Autodesk Inventor part; units mm, degrees
ref_plane "YZ Plane" through (0, 0, 0) normal (1, 0, 0) x (0, 1, 0)
ref_plane "XZ Plane" through (0, 0, 0) normal (0, 1, 0) x (-1, 0, 0)
ref_plane "XY Plane" through (0, 0, 0) normal (0, 0, 1) x (1, 0, 0)
sketch "Skizze1" plane through (0, 0, 0) normal (0, 0, 1) x (1, 0, 0)
  line L0 (0, -1.9) -> (0, 11.4) construction
  line L1 (-7.5, 0) -> (7.5, 0)
  line L2 (7.5, 0) -> (7.5, 9.5)
  line L3 (7.5, 9.5) -> (-7.5, 9.5)
  line L4 (-7.5, 9.5) -> (-7.5, 0)
  circle A0 centre (-7.5, 6.5) radius 1.5
  line L5 (-12.6, 0) -> (12.6, 0)
  line L6 (-4.5, 6.5) -> (-7.5, 6.5) construction
  line L7 (-4.5, 7) -> (-7.5, 7)
  line L8 (-7.5, 6) -> (-4.5, 6)
  arc A1 (-4.5, 6) -> (-4.5, 7) centre (-4.5, 6.5) ccw
  arc A2 (-7.5, 7) -> (-7.5, 6) centre (-7.5, 6.5) ccw
  circle A3 centre (-4.5, 6.5) radius 1
  circle A4 centre (7.5, 6.5) radius 1.5
  line L9 (4.5, 7) -> (7.5, 7)
  line L10 (7.5, 6) -> (4.5, 6)
  arc A5 (4.5, 7) -> (4.5, 6) centre (4.5, 6.5) ccw
  circle A6 centre (4.5, 6.5) radius 1
  point P0 (0, 0)
  point P1 (0, 0)
  point P2 (-7.5, 8)
  point P3 (-7.5, 5)
  point P4 (-6, 6.5)
  point P5 (6, 6.5)
  point P6 (-6.0858, 7)
  point P7 (-5.366, 7)
  point P8 (-5.366, 6)
  point P9 (-6.0858, 6)
  point P10 (7.5, 5)
  point P11 (6.0858, 6)
  point P12 (5.366, 6)
  point P13 (5.366, 7)
  point P14 (6.0858, 7)
  point P15 (7.5, 8)
  dimension "d2" = 3
  dimension "d0" = 15
  dimension "d1" = 9.5
  dimension "d3" = 3
  dimension "d6" = 1
  dimension "d7" = 2
extrude "Extrusion1" add sketch "Skizze1" along normal blind 550 contours L4 A0 L8 A3 L7 L3 L2 A4 L9 A6 L10 L1
sketch "Skizze2" plane through (-7.5, 9.5, 550) normal (0, 1, 0) x (1, 0, 0)
  line L0 (-3, 550) -> (18, 550)
  line L1 (7.5, 660) -> (7.5, -110)
  circle A0 centre (7.5, 515) radius 3
  circle A1 centre (7.5, 515) radius 1.75
  point P0 (7.5, 550)
  dimension "d8" = 6
  dimension "d9" = 3.5
  dimension "d10" = 35
extrude "Extrusion2" cut sketch "Skizze2" against normal blind 6
extrude "Extrusion3" cut sketch "Skizze2" against normal blind 15 contours A1 L1 | L1 A1
chamfer "Fase1" distance 1 angle 45 1 edges at (-3, 9.5, 35)
pattern_linear "Rechteckige Anordnung1" count 13 spacing 40 along (0, 0, 1) of "Extrusion2", "Extrusion3", "Fase1"
equation "\"d4\" = Raillänge"
equation "\"Raillänge\" = 550"
properties part number "MGN15 Linear Rail 550mm"
Geometry check sheet. Reference: the model listing, model coordinates, mm. Give positions to 0.01 mm unless a question says otherwise; leave off trailing zeros. Order: outer loops, then holes, each group sorted by start corner. A loop starts at its lowest first (then second) coordinate and runs counter-clockwise, first axis right, second up. Notation, with made-up numbers: (42, -37.5) - (90, -37.5) arc R37 cw to (90, -0.5) - close; hole circle Ø8 at (63.25, 9). An arc over 180 degrees is marked (long way). Write item = value, one per line. Start each with the question number.
1) Section check A-A (z = 257). Enter the section's corners in (x, y), then the cut area to 3 significant figures.
2) Section check B-B (y = 1.5). Count the separate pieces of the cut face and the enclosed holes in it, then the cut area to 3 significant figures.
3) Scan lines: L1, parallel to X at y = 4.75, z = 275; L2, parallel to Y at x = -6, z = 314.5; L3, parallel to X at y = 1.2, z = 475. Record each from-to range of solid material in increasing order.
4) Gauge pin test, flat ends, axial feed: pin 1 Ø1.5 at (x, z) = (1, 207) entering from -Y; pin 2 Ø1.8 at (x, z) = (1, 436) entering from +Y; pin 3 Ø2 at (y, z) = (6.5, 451) entering from +X. Record the tip position at first contact, or that the pin passes through.
Geometry check:
q1.outline = (-7.5, 0) - (7.5, 0) - (7.5, 5) arc R1.5 cw to (6.09, 6) - (5.37, 6) arc R1 cw (long way) to (5.37, 7) - (6.09, 7) arc R1.5 cw to (7.5, 8) - (7.5, 9.5) - (-7.5, 9.5) - (-7.5, 8) arc R1.5 cw to (-6.09, 7) - (-5.37, 7) arc R1 cw (long way) to (-5.37, 6) - (-6.09, 6) arc R1.5 cw to (-7.5, 5) - close
q1.area = 128 mm2
q2.separate_pieces = 1
q2.enclosed_holes = 13
q2.area = 8,120 mm2
q3.L1 = -7.5 to -3, 3 to 7.5
q3.L2 = 0 to 6, 7 to 9.5
q3.L3 = -7.5 to -1.75, 1.75 to 7.5
q4.pin_1 = 0
q4.pin_2 = 3.5
q4.pin_3 = 6.38
